Geometry: see drawing. Coordinates: mm, zero at the bounding-box minimum. A direction names the side the tool comes from. Coordinates: 2 decimals unless noted, no trailing zeros. Loops run counter-clockwise (first coordinate to the right, second up) from the corner with the lowest first, then second, coordinate; pieces in that order, holes last. Notation, with made-up numbers: (-2.5, -8) -> (23.5, -8) arc R18 ccw to (23.5, -3) -> close; hole circle Ø3 at (81, 55.5). An arc over 180 degrees is marked (long way). Put each result on its own line as item: value. Start each with the question number.
1) Cut plane A-A (y = 7.5). Return the cut outline in (x, z).
2) Cut plane C-C (y = 1.5). Return the cut outline in (x, z), plus the area to 3 significant figures.
3) Material intervals for L1, parallel to Y at x = 7.5, z = 3.1; L2, parallel to Y at x = 6.75, z = 1.05; L3, parallel to X at y = 10, z = 1.2, sorted ascending.
4) Cut plane D-D (z = 1.7). Return the cut outline in (x, y).
5) Set-up query: the marked faces 1 and 2. Return all of +Z, -Z, +X, -X, +Y, -Y with unobstructed straight access to the full face (end or side cutting, diameter ignored); none if empty.
6) Contact query for a flat-ended pin moving along its axis: P1, Ø2, axis at y = 7.5, z = 3, coming from the +X side. Output: stop coordinate, or through.
7) Pull-direction query (X, two-part tool) for the marked faces 3, 4 and 5; classes: pulls with the +X half, pulls with the -X half, needs draft (parallel to the pull), parting line crosses it, or undercut.
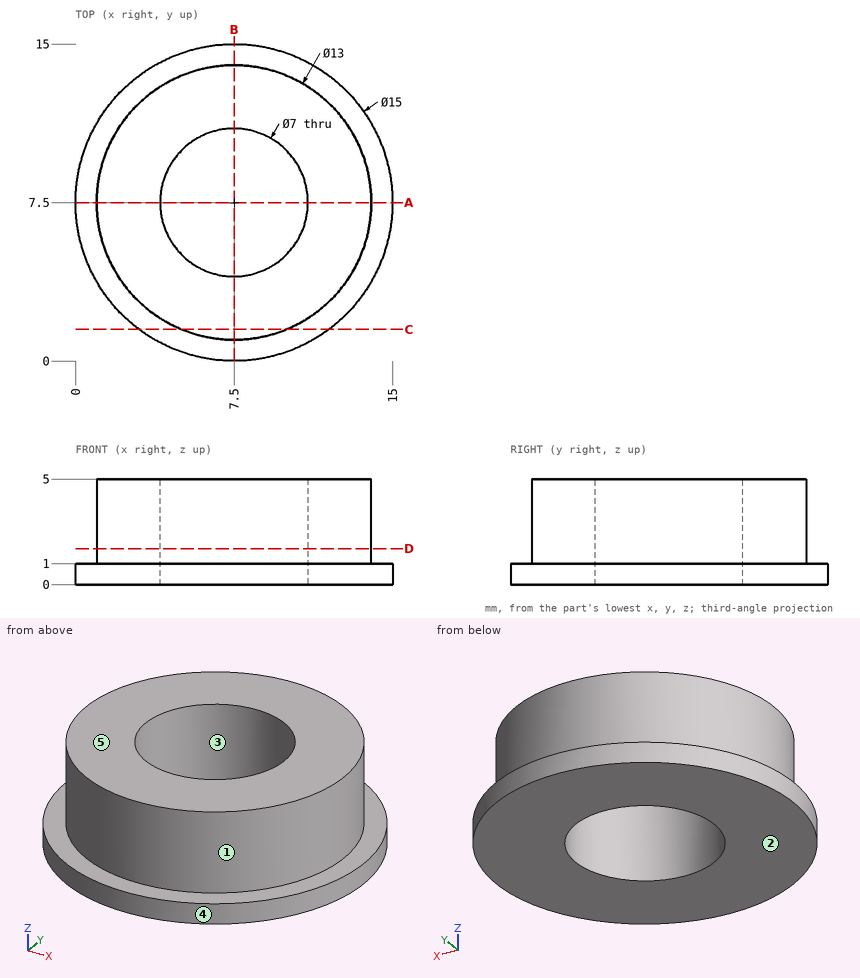
Results found:
1. outline: (0, 0) -> (4, 0) -> (4, 5) -> (1, 5) -> (1, 1) -> (0, 1) -> close; (11, 0) -> (15, 0) -> (15, 1) -> (14, 1) -> (14, 5) -> (11, 5) -> close
2. outline: (3, 0) -> (12, 0) -> (12, 1) -> (10, 1) -> (10, 5) -> (5, 5) -> (5, 1) -> (3, 1) -> close
2. area: 29.0 mm2
3. L1: y = 1 to 4, 11 to 14
3. L2: y = 1.04 to 4.08, 10.92 to 13.96
3. L3: x = 1.5 to 5.05, 9.95 to 13.5
4. outline: circle Ø13 at (7.5, 7.5); hole circle Ø7 at (7.5, 7.5)
5. face 1: +Z
5. face 2: -Z, +X, -X, +Y, -Y
6. P1: stops at x = 14
7. face 3: undercut
7. face 4: parting line crosses it
7. face 5: needs draft
